Geometry check sheet. Reference: the model listing, model coordinates, mm. Face numbers are marked on the shaded views. A direction names the side the tool comes from. Round coordinates to 2 decimals unless told otherwise and drop trailing zeros. Write each loop counter-clockwise with the first axis right and the second up, starting at its lowest first coordinate (ties: lowest second). Pieces come first, ordered by that corner, then holes. Notation, with made-up numbers: M 12,-4.75 L 68,-4.75 A19 cw 68,3.25 Z; hole C -1.5,6 d7. An arc over 180 degrees is marked long. Answer in a Markdown table with one row per item. Add a question column.
from build123d import *

# Parameters (mm, degrees)
SKETCH2_W          = 0.6
SKETCH2_H          = 12
SKETCH3_R          = 1
CUT_EXTRUDE1_DEPTH = 10


with BuildPart() as part:
    # Sweep1: sweep along a path in Sketch1
    with BuildLine(Plane(origin=(0, 0, 0), x_dir=(1, 0, 0), z_dir=(0, 1, 0))) as sweep1_path:
        Line((0, 0), (4, 0))
        Line((4, 0), (5, 1.6))
        Line((5, 1.6), (29.454736631, 1.6))
    # Sketch2 → Sweep1 (sweep)
    with BuildSketch(Plane(origin=(0, 0, 0), x_dir=(0, 0, -1), z_dir=(1, 0, 0))):
        Rectangle(SKETCH2_W, SKETCH2_H)
    sweep(path=sweep1_path.line, transition=Transition.RIGHT)

    # Sketch3 → Cut-Extrude1 (cut)
    with BuildSketch(Plane(origin=(0, 0, -0.3), x_dir=(-1, 0, 0), z_dir=(0, 0, -1))):
        with Locations(Location((-2, 0, 0), (0, 0, 90))):
            Circle(SKETCH3_R)
    extrude(amount=-CUT_EXTRUDE1_DEPTH, mode=Mode.SUBTRACT)


solid = part.part
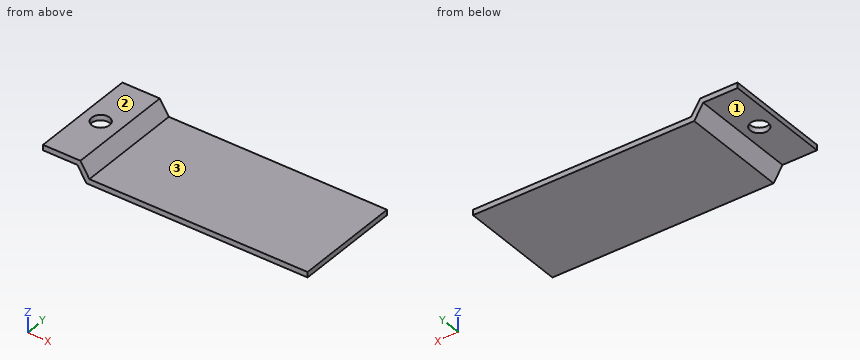
Item 1: Section check D-D, the plane x = 20. Record the boundary of the cut face in (y, z), and give its area (3 significant figures).
Item 2: Section check C-C, the plane y = -5. Record the boundary of the cut face in (x, z), and give its area (3 significant figures).
Item 3: Scan lines: probe 1 along Z at (x, y) = (26, 2.25); probe 2 along X at (y, z) = (0, 0.15); probe 3 along Z at (x, y) = (2.5, 4.75). Record each from-to range of solid material in increasing order. Write a range as from..to.
Item 4: Section check B-B, the plane y = 0. Record the boundary of the cut face in (x, z).
Item 5: Gauge pin test, flat ends, axial feed: pin 1 Ø5 at (x, y) = (14.5, 4) entering from +Z; pin 2 Ø1 at (x, z) = (14.5, -1) entering from -Y; pin 3 Ø4 at (x, y) = (2, 2.5) entering from -Z; pin 4 Ø1.8 at (x, y) = (2, 0) entering from +Z. Record the tip position at first contact, or that the pin passes through.
Item 6: Access from +Z, -Z, +X, -X, +Y, -Y to the whole of each face (thin tool, end or side, straight path). Record for the marked faces 1, 2 and 3.
Item 7: Section check A-A, the plane x = 2. Record the boundary of the cut face in (y, z).
Result sheet:
| question | item | result |
|---|---|---|
| 1 | outline | M -6,-1.9 L 6,-1.9 L 6,-1.3 L -6,-1.3 Z |
| 1 | area | 7.20 mm^2 |
| 2 | outline | M 0,-0.3 L 3.83,-0.3 L 4.83,-1.9 L 29.45,-1.9 L 29.45,-1.3 L 5.17,-1.3 L 4.17,0.3 L 0,0.3 Z |
| 2 | area | 18.2 mm^2 |
| 3 | probe 1 | z = -1.9..-1.3 |
| 3 | probe 2 | x = 0..1, 3..4.26 |
| 3 | probe 3 | z = -0.3..0.3 |
| 4 | outline | M 0,-0.3 L 1,-0.3 L 1,0.3 L 0,0.3 Z; M 3,-0.3 L 3.83,-0.3 L 4.83,-1.9 L 29.45,-1.9 L 29.45,-1.3 L 5.17,-1.3 L 4.17,0.3 L 3,0.3 Z |
| 5 | pin 1 | stops at z = -1.3 |
| 5 | pin 2 | stops at y = -6 |
| 5 | pin 3 | stops at z = -0.57 |
| 5 | pin 4 | passes through |
| 6 | face 1 | -Z, -X, +Y, -Y |
| 6 | face 2 | +Z, +X, -X, +Y, -Y |
| 6 | face 3 | +Z, +X, +Y, -Y |
| 7 | outline | M -6,-0.3 L -1,-0.3 L -1,0.3 L -6,0.3 Z; M 1,-0.3 L 6,-0.3 L 6,0.3 L 1,0.3 Z |
